Work out the finished part from the listing and answer in its coordinate system (mm). A direction names the side the tool comes from. Give positions to 0.01 mm unless a question says otherwise; leave off trailing zeros. Loops run counter-clockwise (first coordinate to the right, second up) from the corner with the lowest first, then second, coordinate; pieces in that order, holes last. Notation, with made-up numbers: M -12,66.5 L 44,66.5 A21 ccw 44,93.5 Z; hole C 81,28 d5. An arc over 180 degrees is marked long. Write item = value, one per line. Start each with the question number.
1. Section C-C on z = 653.5 is taken. Determine the outline of the cut face in (x, y).
2. Consider L1, parallel to X at y = 48, z = 620; L2, parallel to Y at x = 14, z = 85; L3, parallel to X at y = 1, z = 218.5. Determine where each line is inside the solid, lowest interval first. Write a range as [from, to].
3. For faces 4 (the face through (25.572, 46.056, 217.013)), 5 (the face through (29, 42, 493)), 6 (the face through (0, 0, 0)), 7 (the face through (1, 50, 493)), 8 (the face through (-30, 42, 493)), determine the directions among +Z, -Z, +X, -X, +Y, -Y from which every point of the face is accessible in a straight line to the end or side of a thin tool.
4. Flat-ended cylindrical pins translate along their axes: pin 1 Ø10 at (y, z) = (-28.5, 617.5) entering from -X; pin 2 Ø15.5 at (x, z) = (25, 380) entering from +Y; pin 3 Ø12 at (x, y) = (12, -16.5) entering from +Z; pin 4 Ø8 at (y, z) = (-10, 691.5) entering from +X. Find the tip coordinate at first contact, or state that the pin passes through.
5. The mould has two halves that part along X. Classify faces 1 (the face through (-4, 1, 493)), 2 (the face through (4, -1, 493)), 3 (the face through (25.572, 46.056, 367.013)): released by +X, released by -X, zero draft, split by the parting line, or undercut.
6. Section A-A on z = 230 is taken. Determine the outline of the cut face in (x, y), plus the area to 3 significant figures.
7. Section D-D on y = -16 is taken. Determine the outline of the cut face in (x, z).
8. Section B-B on x = -25 is taken. Determine the outline of the cut face in (y, z).
```python
from build123d import *

# Parameters (mm, degrees)
BOSS_EXTRUDE1_DEPTH = 1000
FILLET1_R           = 5
SKETCH2_R           = 13
CUT_EXTRUDE1_DEPTH  = 10
SKETCH3_R           = 13
CUT_EXTRUDE2_DEPTH  = 10
SKETCH4_W           = 10
SKETCH4_H           = 30
BOSS_EXTRUDE2_DEPTH = 146
SKETCH6_R           = 15
BOSS_EXTRUDE4_DEPTH = 10
SPLIT1_START        = 495
SPLIT1_OUTLINE_R    = 15
SPLIT1_DEPTH        = 10
SPLIT2_START        = 495
SPLIT2_OUTLINE_R    = 15
SPLIT2_DEPTH        = 10


# Read off the part's stored shape, not the designer's step: Split1, Split2
with BuildPart() as part:
    # Sketch1 → Boss-Extrude1 (new body)
    with BuildSketch(Plane.XY):
        Polygon((-50, 42), (-4, 42), (-4, -42), (-50, -42), (-50, -50), (50, -50), (50, -42), (4, -42), (4, 42), (50, 42), (50, 50), (-50, 50), align=None)
    extrude(amount=BOSS_EXTRUDE1_DEPTH)

    # Fillet1
    fillet1_edges = [part.edges().sort_by_distance(p)[0] for p in [
        (4, 42, 500),
        (4, -42, 500),
        (-4, -42, 500),
        (-4, 42, 500),
    ]]
    fillet(fillet1_edges, radius=FILLET1_R)

    # Sketch2 → Cut-Extrude1 (cut)
    with BuildSketch(Plane(origin=(0, 50, 0), x_dir=(1, 0, 0), z_dir=(0, 1, 0))):
        with Locations(Location((25, -770, 0), (0, 0, 270))):
            Circle(SKETCH2_R)
        with Locations(Location((-25, -770, 0), (0, 0, 270))):
            Circle(SKETCH2_R)
        with Locations(Location((25, -230, 0), (0, 0, 270))):
            Circle(SKETCH2_R)
        with Locations(Location((-25, -230, 0), (0, 0, 270))):
            Circle(SKETCH2_R)
    extrude(amount=-CUT_EXTRUDE1_DEPTH, mode=Mode.SUBTRACT)

    # Sketch3 → Cut-Extrude2 (cut)
    with BuildSketch(Plane(origin=(0, 50, 0), x_dir=(1, 0, 0), z_dir=(0, 1, 0))):
        with Locations(Location((-25, -620, 0), (0, 0, 270))):
            Circle(SKETCH3_R)
        with Locations(Location((25, -620, 0), (0, 0, 270))):
            Circle(SKETCH3_R)
        with Locations(Location((25, -380, 0), (0, 0, 270))):
            Circle(SKETCH3_R)
        with Locations(Location((-25, -380, 0), (0, 0, 270))):
            Circle(SKETCH3_R)
    extrude(amount=-CUT_EXTRUDE2_DEPTH, mode=Mode.SUBTRACT)

    # Sketch4 → Boss-Extrude2 (add)
    with BuildSketch(Plane(origin=(4, 0, 0), x_dir=(0, 0, -1), z_dir=(1, 0, 0))):
        with Locations((-500, -5.392878346)):
            Rectangle(SKETCH4_W, SKETCH4_H)
    boss_extrude2 = extrude(amount=BOSS_EXTRUDE2_DEPTH)

    # Sketch6 → Boss-Extrude4 (add)
    with BuildSketch(Plane.XY.offset(505)):
        Polygon((150, 9.607121654), (150, -70.392878346), (180, -70.392878346), (220, -20.392878346), (220, 9.607121654), align=None)
        with Locations((185, -10.392878346)):
            Circle(SKETCH6_R, mode=Mode.SUBTRACT)
    boss_extrude4 = extrude(amount=-BOSS_EXTRUDE4_DEPTH)

    # Mirror1: Boss-Extrude2, Boss-Extrude4 across plane
    add(boss_extrude2.mirror(Plane(origin=(0, 0, 0), x_dir=(0, 0, 1), z_dir=(1, 0, 0))))
    add(boss_extrude4.mirror(Plane(origin=(0, 0, 0), x_dir=(0, 0, 1), z_dir=(1, 0, 0))))

    # Split1 outline → Split1 (cut)
    with BuildSketch(Plane.XY.offset(SPLIT1_START)):
        Polygon((-150, -20.392878346), (-4, -20.392878346), (-4, 9.607121654), (-220, 9.607121654), (-220, -20.392878346), (-180, -70.392878346), (-150, -70.392878346), align=None)
        with Locations((-185, -10.392878346)):
            Circle(SPLIT1_OUTLINE_R, mode=Mode.SUBTRACT)
    extrude(amount=SPLIT1_DEPTH, mode=Mode.SUBTRACT)

    # Split2 outline → Split2 (cut)
    with BuildSketch(Plane.XY.offset(SPLIT2_START)):
        Polygon((4, -20.392878346), (150, -20.392878346), (150, -70.392878346), (180, -70.392878346), (220, -20.392878346), (220, 9.607121654), (4, 9.607121654), align=None)
        with Locations((185, -10.392878346)):
            Circle(SPLIT2_OUTLINE_R, mode=Mode.SUBTRACT)
    extrude(amount=SPLIT2_DEPTH, mode=Mode.SUBTRACT)


solid = part.part
```
Verdict:
q1.outline = M -50,-50 L 50,-50 L 50,-42 L 9,-42 A5 cw 4,-37 L 4,37 A5 cw 9,42 L 50,42 L 50,50 L -50,50 L -50,42 L -9,42 A5 cw -4,37 L -4,-37 A5 cw -9,-42 L -50,-42 Z
q2.L1 = [-50, -38], [-12, 12], [38, 50]
q2.L2 = [-50, -42], [42, 50]
q2.L3 = [-4, 4]
q3.face_4 = +Y
q3.face_5 = +Z, -Z, +X
q3.face_6 = -Z, +X, -X, +Y, -Y
q3.face_7 = +Z, -Z, +X, -X, +Y
q3.face_8 = +Z, -Z, -X
q4.pin_1 = -4
q4.pin_2 = -42
q4.pin_3 = through
q4.pin_4 = 4
q5.face_1 = released by -X
q5.face_2 = released by +X
q5.face_3 = undercut
q6.outline = M -50,-50 L 50,-50 L 50,-42 L 9,-42 A5 cw 4,-37 L 4,37 A5 cw 9,42 L 12,42 L 12,50 L -12,50 L -12,42 L -9,42 A5 cw -4,37 L -4,-37 A5 cw -9,-42 L -50,-42 Z; M -50,42 L -38,42 L -38,50 L -50,50 Z; M 38,42 L 50,42 L 50,50 L 38,50 Z
q6.area = 1,880 mm2
q7.outline = M -4,0 L 4,0 L 4,1000 L -4,1000 Z
q8.outline = M -50,0 L -42,0 L -42,1000 L -50,1000 Z; M 42,0 L 50,0 L 50,217 L 42,217 Z; M 42,243 L 50,243 L 50,367 L 42,367 Z; M 42,393 L 50,393 L 50,607 L 42,607 Z; M 42,633 L 50,633 L 50,757 L 42,757 Z; M 42,783 L 50,783 L 50,1000 L 42,1000 Z
